Source: CAD feature listing. Evaluate the final solid. Frame: model axes, mm. A direction names the side the tool comes from. Round coordinates to 2 decimals unless told otherwise and drop trailing zeros. Order: outer loops, then holes, each group sorted by start corner. A loop starts at its lowest first (then second) coordinate and runs counter-clockwise, first axis right, second up. Notation, with made-up numbers: (48, 2) -> (60, 2) arc R23 ccw to (60, 17) -> close; hole circle Ø8 at (81, -32.75). An arc over 180 degrees is marked (long way). One line per item, written item: value. Start each with the question number.
1) Section A-A (x = 3). Return the cut outline in (y, z), and give its area (3 significant figures).
2) Pin query (flat end, axial travel): P1, Ø1, axis at x = -24.5, z = 1.5, coming from the -Y side; P2, Ø4, axis at x = 5.5, y = -25.5, coming from the -Z side; P3, Ø0.6, axis at x = 24, z = 0.5, coming from the +Y side. Return the tip coordinate at first contact, or that it passes through.
3) Reachability of faces 1 (the face through (-27, 5.57, 0.99)), 2 (the face through (11, 21, 1)) from +Z, -Z, +X, -X, +Y, -Y: full face, straight path, thin tool, end or side. Return the list, or none.
4) Section B-B (z = 0.5). State how many separate pieces and enclosed holes the cut face has, and give its area (3 significant figures).
5) Ray query, L1, parallel to Y at x = -25.5, z = 1.35; L2, parallel to Y at x = 5.5, z = 0.65; L3, parallel to X at y = 26.5, z = 1.7. Return the intervals inside material, ascending.
6) Mould query, pull axis X, two halves, no side actions, for faces 3 (the face through (-7, -37, 1)), 4 (the face through (-26.61, -24.49, 0.99)), 5 (the face through (14, -43, 1)). Classes: pulls with the +X half, pulls with the -X half, needs draft (parallel to the pull), parting line crosses it, or undercut.
7) Section D-D (y = 21). Return the cut outline in (x, z).
8) Section C-C (y = 5.5). Return the cut outline in (x, z).
```python
from build123d import *

# Parameters (mm, degrees)
F0_R     = 1.5
F0_R_2   = 11
F0_R_3   = 2
F1_DEPTH = 2
F2_SIZE  = 5
F3_W     = 38
F3_H     = 12
F4_DEPTH = 2
F5_R     = 2
F6_DEPTH = 25
F7_R     = 5


with BuildPart() as f1:
    # F0 (on Top) → F1 (new body)
    with BuildSketch(Plane.XY):
        Polygon((-31, -31), (31, -31), (31, 11), (11, 11), (11, 31), (-31, 31), align=None)
        with Locations((-25.5, -25.5)):
            Circle(F0_R, mode=Mode.SUBTRACT)
        with Locations((-10, -10)):
            Circle(F0_R_2, mode=Mode.SUBTRACT)
        with Locations((5.5, -25.5)):
            Circle(F0_R, mode=Mode.SUBTRACT)
        with Locations((21, -17)):
            Circle(F0_R_3, mode=Mode.SUBTRACT)
        with Locations((-25.5, 5.5)):
            Circle(F0_R, mode=Mode.SUBTRACT)
        with Locations((-10, 21)):
            Circle(F0_R_3, mode=Mode.SUBTRACT)
        with Locations((5.5, 5.5)):
            Circle(F0_R, mode=Mode.SUBTRACT)
    extrude(amount=F1_DEPTH)

    # F2
    f2_edges = [f1.edges().sort_by_distance(p)[0] for p in [
        (-31, -31, 1),
    ]]
    chamfer(f2_edges, length=F2_SIZE)

    # F3 (on face) → F4 (join)
    with BuildSketch(Plane.XY.offset(2)):
        with Locations((12, -37)):
            Rectangle(F3_W, F3_H)
    extrude(amount=-F4_DEPTH)

    # F5 (on face) → F6 (cut)
    with BuildSketch(Plane.XY.offset(2)):
        with Locations((3, -36)):
            Circle(F5_R)
    extrude(amount=-F6_DEPTH, mode=Mode.SUBTRACT)

    # F7
    f7_edges = [f1.edges().sort_by_distance(p)[0] for p in [
        (-7, -43, 1),
        (-7, -31, 1),
    ]]
    fillet(f7_edges, radius=F7_R)


solid = f1.part
```
Findings:
1. outline: (-43, 0) -> (-38, 0) -> (-38, 2) -> (-43, 2) -> close; (-34, 0) -> (31, 0) -> (31, 2) -> (-34, 2) -> close
1. area: 140 mm2
2. P1: y = -31
2. P2: z = 0
2. P3: y = 11
3. face 1: +Z, -Z
3. face 2: +Z, -Z, +X, +Y
4. separate pieces: 1
4. enclosed holes: 8
4. area: 3,440 mm2
5. L1: -31 to -27, -24 to 4, 7 to 31
5. L2: -43 to -27, -24 to 4, 7 to 31
5. L3: -31 to 11
6. face 3: pulls with the -X half
6. face 4: undercut
6. face 5: needs draft
7. outline: (-31, 0) -> (-12, 0) -> (-12, 2) -> (-31, 2) -> close; (-8, 0) -> (11, 0) -> (11, 2) -> (-8, 2) -> close
8. outline: (-31, 0) -> (-27, 0) -> (-27, 2) -> (-31, 2) -> close; (-24, 0) -> (4, 0) -> (4, 2) -> (-24, 2) -> close; (7, 0) -> (31, 0) -> (31, 2) -> (7, 2) -> close
